from build123d import *

# Parameters (mm, degrees)
F1_DEPTH       = 5
F3_D           = 2.5
F3_CBORE_D     = 6.5
F3_CBORE_DEPTH = 3


with BuildPart() as f1:
    # F0 (on Top) → F1 (new body)
    with BuildSketch(Plane.XY):
        with BuildLine():
            Line((-3.4954430428, 12.0013281738), (-17.2336879396, 8))
            ThreePointArc((-17.2336879396, 8), (-19, 0), (-17.2336879396, -8))
            Line((-17.2336879396, -8), (-3.4954430428, -12.0013281738))
            ThreePointArc((-3.4954430428, -12.0013281738), (0, -12.5), (3.4954430428, -12.0013281738))
            Line((3.4954430428, -12.0013281738), (17.2336879396, -8))
            ThreePointArc((17.2336879396, -8), (19, 0), (17.2336879396, 8))
            Line((17.2336879396, 8), (3.4954430428, 12.0013281738))
            ThreePointArc((3.4954430428, 12.0013281738), (0, 12.5), (-3.4954430428, 12.0013281738))
        make_face()
    extrude(amount=F1_DEPTH)

    # F3 (through all)
    with Locations(Plane.XY.offset(5)):
        with Locations((-9.5, 0), (0, 8), (9.5, 0), (0, -8), (-16.5, 0), (16.5, 0)):
            CounterBoreHole(F3_D / 2, F3_CBORE_D / 2, F3_CBORE_DEPTH)


solid = f1.part
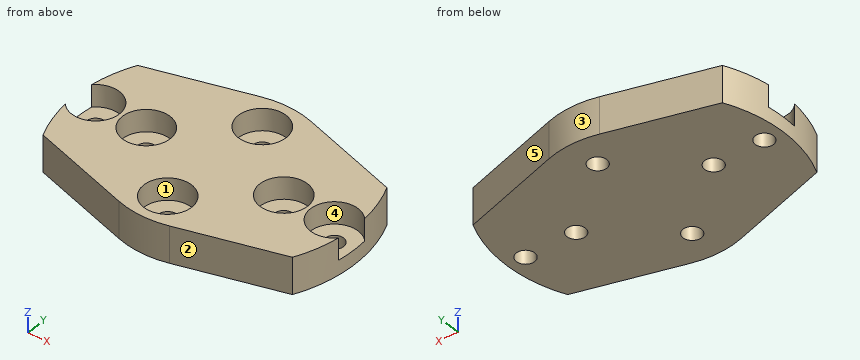
Verification items for the finished model (mm, model axes). Face numbers are marked on the shaded views. A direction names the side the tool comes from. Coordinates: 2 decimals unless noted, no trailing zeros. Loops run counter-clockwise (first coordinate to the right, second up) from the corner with the lowest first, then second, coordinate; pieces in that order, holes last. Notation, with made-up numbers: (8, -35.75) -> (20, -35.75) arc R21 cw to (20, -14.75) -> close; hole circle Ø6 at (86.25, -36). An arc over 180 degrees is marked (long way). Answer as a JSON object with one key per item and string values. Group by question number.
Item 1: Sectioned sample at C-C on y = -8.75. Record the boundary of the cut face in (x, z).
Item 2: Depth check by flat-ended pin: pin 1 (3 mm diameter, centred on x = -16, y = -1.5, fed in from +Z); pin 2 (2 mm diameter, centred on x = -10.5, z = 1, fed in from +Y). Enter the tip coordinate at first touch or a pass-through.
Item 3: Tool access check on the marked faces 1 and 2. Record the directions out of +Z, -Z, +X, -X, +Y, -Y that give a thin tool (end or side, any length) a straight path to the whole face; none if there is none.
Item 4: Mould release check, pull along X, two halves, no side actions. Record for the marked faces 3, 4 and 5: +X half, -X half, draft (parallel to the pull), parting line (faces both ways), or undercut.
Item 5: Sectioned sample at D-D on x = 16.5. Record the boundary of the cut face in (y, z), plus the area to 3 significant figures.
Item 6: Scan lines: probe 1 along Y at (x, z) = (0, 1.2); probe 2 along Y at (x, z) = (0, 3.4); probe 3 along Z at (x, y) = (16, -1.75). Record each from-to range of solid material in increasing order.
Item 7: Sectioned sample at A-A on x = 0. Record the boundary of the cut face in (y, z).
Item 8: Sectioned sample at B-B on z = 1. Record the boundary of the cut face in (x, y), plus the area to 3 significant figures.
Evaluation:
{
 "1": {"outline": "(-14.66, 0) -> (-1, 0) -> (-1, 2) -> (-3.16, 2) -> (-3.16, 5) -> (-14.66, 5) -> close; (1, 0) -> (14.66, 0) -> (14.66, 5) -> (3.16, 5) -> (3.16, 2) -> (1, 2) -> close"},
 "2": {"pin 1": "stops at z = 2", "pin 2": "stops at y = 10.25"},
 "3": {"face 1": "+Z", "face 2": "+Z, -Z, +X, -Y"},
 "4": {"face 3": "parting line", "face 4": "undercut", "face 5": "+X half"},
 "5": {"outline": "(-8.21, 0) -> (-1.25, 0) -> (-1.25, 2) -> (-3.25, 2) -> (-3.25, 5) -> (-8.21, 5) -> close; (1.25, 0) -> (8.21, 0) -> (8.21, 5) -> (3.25, 5) -> (3.25, 2) -> (1.25, 2) -> close", "area": "57.6 mm²"},
 "6": {"probe 1": "y = -12.5 to -9.25, -6.75 to 6.75, 9.25 to 12.5", "probe 2": "y = -12.5 to -11.25, -4.75 to 4.75, 11.25 to 12.5", "probe 3": "z = 0 to 2"},
 "7": {"outline": "(-12.5, 0) -> (-9.25, 0) -> (-9.25, 2) -> (-11.25, 2) -> (-11.25, 5) -> (-12.5, 5) -> close; (-6.75, 0) -> (6.75, 0) -> (6.75, 2) -> (4.75, 2) -> (4.75, 5) -> (-4.75, 5) -> (-4.75, 2) -> (-6.75, 2) -> close; (9.25, 0) -> (12.5, 0) -> (12.5, 5) -> (11.25, 5) -> (11.25, 2) -> (9.25, 2) -> close"},
 "8": {"outline": "(-17.23, -8) -> (-3.5, -12) arc R12.5 ccw to (3.5, -12) -> (17.23, -8) arc R19 ccw to (17.23, 8) -> (3.5, 12) arc R12.5 ccw to (-3.5, 12) -> (-17.23, 8) arc R19 ccw to start; hole circle Ø2.5 at (-16.5, 0); hole circle Ø2.5 at (-9.5, 0); hole circle Ø2.5 at (0, -8); hole circle Ø2.5 at (0, 8); hole circle Ø2.5 at (9.5, 0); hole circle Ø2.5 at (16.5, 0)", "area": "731 mm²"}
}
